Verification items for the finished model (mm, model axes). Face numbers are marked on the shaded views. A direction names the side the tool comes from. Coordinates: 2 decimals unless noted, no trailing zeros. Write each loop counter-clockwise with the first axis right and the second up, starting at its lowest first coordinate (ties: lowest second). Pieces come first, ordered by that corner, then holes.
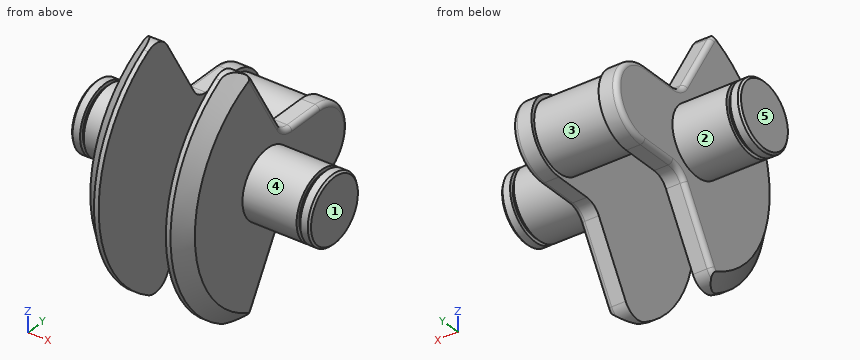
```python
from build123d import *

# Parameters (mm, degrees)
BOSS_EXTRUDE1_DEPTH      = 10
CHAMFER1_SIZE            = 7.5
FILLET1_R                = 2.5
BOSS_EXTRUDE2_DEPTH      = 10
CHAMFER2_SIZE            = 7.5
FILLET2_R                = 2.5
SKETCH3_R                = 18
BOSS_EXTRUDE3_DEPTH      = 18
SKETCH4_R                = 18
BOSS_EXTRUDE4_DEPTH      = 36
SKETCH5_W                = 2
SKETCH5_H                = 2
CHAMFER3_SIZE            = 1
CHAMFER3_OF_MIRROR1_SIZE = 1


with BuildPart() as part:
    # Sketch1 → Boss-Extrude1 (new body)
    with BuildSketch(Plane(origin=(18, 0, 0), x_dir=(0, 0, -1), z_dir=(1, 0, 0))):
        with BuildLine():
            Line((-25, -28.886751346), (-58.693575035, -48.339745962))
            ThreePointArc((-58.693575035, -48.339745962), (-63.352833298, -54.411809549), (-62.353829072, -62))
            ThreePointArc((-62.353829072, -62), (0, -98), (62.353829072, -62))
            ThreePointArc((62.353829072, -62), (63.352833298, -54.411809549), (58.693575035, -48.339745962))
            Line((58.693575035, -48.339745962), (25, -28.886751346))
            ThreePointArc((25, -28.886751346), (21.339745962, -25.226497308), (20, -20.226497308))
            Line((20, -20.226497308), (20, 0))
            ThreePointArc((20, 0), (0, 20), (-20, 0))
            Line((-20, 0), (-20, -20.226497308))
            ThreePointArc((-20, -20.226497308), (-21.339745962, -25.226497308), (-25, -28.886751346))
        make_face()
    extrude(amount=BOSS_EXTRUDE1_DEPTH)

    # Chamfer1
    # the kernel refuses this chamfer: 7.5 mm, written as the material it takes off along each edge
    with BuildSketch(Plane(origin=(28, -26, 0), x_dir=(0, -0.2527522173180771, 0.9675310416936479), z_dir=(0, 0.9675310416936479, 0.2527522173180771))) as chamfer1_piece_1:
        Polygon((72, -CHAMFER1_SIZE), (72 - CHAMFER1_SIZE, 0), (72, 0), align=None)
    revolve(axis=Axis((28, -26, 0), (1, 0, 0)), revolution_arc=150.719131607, mode=Mode.SUBTRACT)

    # Fillet1
    fillet1_edges = [part.edges().sort_by_distance(p)[0] for p in [
        (28, -48.810655601, -59.432445857),
        (28, -38.613248654, -41.846787517),
        (28, -25.226497308, -21.339745962),
        (28, -10.113248654, -20),
        (28, -48.810655601, 59.432445857),
        (28, -38.613248654, 41.846787517),
        (28, -25.226497308, 21.339745962),
        (28, -10.113248654, 20),
        (28, 20, 0),
    ]]
    fillet(fillet1_edges, radius=FILLET1_R)



with BuildPart() as body_2:
    # Sketch2 → Boss-Extrude2 (new body)
    with BuildSketch(Plane(origin=(-18, 0, 0), x_dir=(0, 0, -1), z_dir=(1, 0, 0))):
        with BuildLine():
            Line((20, -20.226497308), (20, 0))
            ThreePointArc((20, 0), (0, 20), (-20, 0))
            Line((-20, 0), (-20, -20.226497308))
            ThreePointArc((-20, -20.226497308), (-21.339745962, -25.226497308), (-25, -28.886751346))
            Line((-25, -28.886751346), (-58.693575035, -48.339745962))
            ThreePointArc((-58.693575035, -48.339745962), (-63.352833298, -54.411809549), (-62.353829072, -62))
            ThreePointArc((-62.353829072, -62), (0, -98), (62.353829072, -62))
            ThreePointArc((62.353829072, -62), (63.352833298, -54.411809549), (58.693575035, -48.339745962))
            Line((58.693575035, -48.339745962), (25, -28.886751346))
            ThreePointArc((25, -28.886751346), (21.339745962, -25.226497308), (20, -20.226497308))
        make_face()
    extrude(amount=-BOSS_EXTRUDE2_DEPTH)

    # Chamfer2
    # the kernel refuses this chamfer: 7.5 mm, written as the material it takes off along each edge
    with BuildSketch(Plane(origin=(-28, -26, 0), x_dir=(0, -0.25275221731807723, 0.9675310416936479), z_dir=(0, 0.9675310416936479, 0.25275221731807723))) as chamfer2_piece_1:
        Polygon((72, CHAMFER2_SIZE), (72 - CHAMFER2_SIZE, 0), (72, 0), align=None)
    revolve(axis=Axis((-28, -26, 0), (1, 0, 0)), revolution_arc=150.719131607, mode=Mode.SUBTRACT)

    # Fillet2
    fillet2_edges = [body_2.edges().sort_by_distance(p)[0] for p in [
        (-28, -48.810655601, -59.432445857),
        (-28, -38.613248654, -41.846787517),
        (-28, -25.226497308, -21.339745962),
        (-28, -10.113248654, -20),
        (-28, -48.810655601, 59.432445857),
        (-28, -38.613248654, 41.846787517),
        (-28, -25.226497308, 21.339745962),
        (-28, -10.113248654, 20),
        (-28, 20, 0),
    ]]
    fillet(fillet2_edges, radius=FILLET2_R)


with BuildPart() as part_1:
    add(part.part)

    add(body_2.part)  # Boss-Extrude3 merges body 2
    # Sketch3 → Boss-Extrude3 (add, symmetric)
    with BuildSketch(Plane(origin=(0, 0, 0), x_dir=(0, 0, -1), z_dir=(1, 0, 0))):
        Circle(SKETCH3_R)
    extrude(amount=BOSS_EXTRUDE3_DEPTH, both=True)

    # Sketch4 → Boss-Extrude4 (add)
    with BuildSketch(Plane(origin=(28, 0, 0), x_dir=(0, 0, -1), z_dir=(1, 0, 0))):
        with Locations((0, -38)):
            Circle(SKETCH4_R)
    boss_extrude4 = extrude(amount=BOSS_EXTRUDE4_DEPTH)

    # Sketch5 → Cut-Revolve1 (revolve, cut)
    with BuildSketch(Plane.XY, mode=Mode.PRIVATE) as cut_revolve1_sk:
        with Locations((58, -21)):
            Rectangle(SKETCH5_W, SKETCH5_H)
    cut_revolve1 = revolve(cut_revolve1_sk.sketch.rotate(Axis((64, -38, 0), (-1, 0, 0)), 90), axis=Axis((64, -38, 0), (-1, 0, 0)), mode=Mode.SUBTRACT)

    # Chamfer3
    chamfer3_edges = [part_1.edges().sort_by_distance(p)[0] for p in [
        (64, -38, 18),
    ]]
    chamfer(chamfer3_edges, length=CHAMFER3_SIZE)

    # Mirror1: Boss-Extrude4, Cut-Revolve1 across plane
    add(boss_extrude4.mirror(Plane(origin=(0, 0, 0), x_dir=(0, 0, 1), z_dir=(1, 0, 0))))
    add(cut_revolve1.mirror(Plane(origin=(0, 0, 0), x_dir=(0, 0, 1), z_dir=(1, 0, 0))), mode=Mode.SUBTRACT)

    # Chamfer3 of Mirror1
    chamfer3_of_mirror1_edges = [part_1.edges().sort_by_distance(p)[0] for p in [
        (-64, -38, 18),
    ]]
    chamfer(chamfer3_of_mirror1_edges, length=CHAMFER3_OF_MIRROR1_SIZE)


solid = part_1.part
```
1. Sectioned sample at B-B, the plane y = -8. Record the boundary of the cut face in (x, z), and give its area (3 significant figures).
2. Tool access check on the marked faces 1 and 2. Record the directions out of +Z, -Z, +X, -X, +Y, -Y that give a thin tool (end or side, any length) a straight path to the whole face; none if there is none.
3. Draft check along X on the marked faces 3, 4 and 5. Enter one of: pulls with the +X half, pulls with the -X half, needs draft (parallel to the pull), parting line crosses it, or undercut.
4. Gauge pin test, flat ends, axial feed: P1, Ø12, axis at y = -46, z = -40.5, coming from the -X side; P2, Ø5, axis at x = 22.5, y = -25, coming from the +Z side; P3, Ø8, axis at x = 20.5, y = -13, coming from the +Z side. Record the tip position at first contact, or that the pin passes through.
5. Material ranges on L1, parallel to X at y = -62, z = -12; L2, parallel to Y at x = -47.5, z = -1; L3, parallel to X at y = -26.5, z = -20.5, recorded low to high.
6. Sectioned sample at A-A, the plane x = -6. Record the boundary of the cut face in (y, z), and give its area (3 significant figures).
Outcome:
1. outline: (-28, -17.5) arc R2.5 ccw to (-25.5, -20) - (-18, -20) - (-18, -16.12) - (18, -16.12) - (18, -20) - (25.5, -20) arc R2.5 ccw to (28, -17.5) - (28, 17.5) arc R2.5 ccw to (25.5, 20) - (18, 20) - (18, 16.12) - (-18, 16.12) - (-18, 20) - (-25.5, 20) arc R2.5 ccw to (-28, 17.5) - close
1. area: 1,960 mm2
2. face 1: +Z, -Z, +X, +Y, -Y
2. face 2: -X
3. face 3: undercut
3. face 4: needs draft
3. face 5: pulls with the -X half
4. P1: stops at x = -28
4. P2: stops at z = 23.14
4. P3: stops at z = 20
5. L1: x = -28 to -18, 18 to 28
5. L2: y = -55.97 to -20.03
5. L3: x = -27.74 to -18, 18 to 27.74
6. outline: circle Ø36 at (0, 0)
6. area: 1,020 mm2
